Design review of the part built by this model. Coordinates are the model's own, in mm. Round coordinates to 2 decimals unless told otherwise and drop trailing zeros. One line per item, written item: value. Start each with the question number.
Item 1: We need section A-A (y = 0.9). State how many separate pieces and enclosed holes the cut face has, then the cut area to 3 significant figures.
Item 2: For line 1 along X through (y, z) = (1.3, 60); line 2 along Z through (x, y) = (-52.5, 1.05); line 3 along Z through (x, y) = (51.5, 0.1), list the stretches that pass through material, from the lowest coordinate up.
Item 3: Clearance check with a flat-ended pin moving along its axis: pin 1 (3.5 mm diameter, centred on x = 35, z = -60, fed in from -Y). State where the tip first meets the part, or that it passes through.
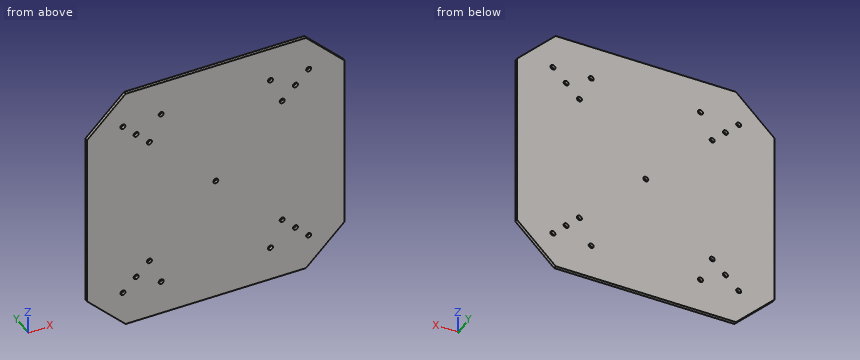
from build123d import *

# Parameters (mm, degrees)
BOSS_EXTRUDE1_DEPTH  = 2
M3_CLEARANCE_HOLE1_D = 3.2
M3_CLEARANCE_HOLE2_D = 3.2


with BuildPart() as part:
    # Sketch1 → Boss-Extrude1 (new body)
    with BuildSketch(Plane(origin=(0, 0, 0), x_dir=(1, 0, 0), z_dir=(0, 1, 0))):
        Polygon((-57.751262658, 82.5), (-82.5, 57.751262658), (-82.5, -57.751262658), (-57.751262658, -82.5), (57.751262658, -82.5), (82.5, -57.751262658), (82.5, 57.751262658), (57.751262658, 82.5), align=None)
    extrude(amount=BOSS_EXTRUDE1_DEPTH)

    # M3 Clearance Hole1 (through all)
    with Locations(Plane(origin=(0, 0, 0), x_dir=(-1, 0, 0), z_dir=(0, -1, 0))):
        with Locations((42.548466863, -42.548466863), (59.519029611, 59.519029611), (51.033748237, 51.033748237), (42.548466863, 42.548466863), (-59.519029611, -59.519029611), (-51.033748237, -51.033748237), (-42.548466863, -42.548466863), (-59.519029611, 59.519029611), (-51.033748237, 51.033748237), (-42.548466863, 42.548466863), (59.519029611, -59.519029611), (51.033748237, -51.033748237)):
            Hole(M3_CLEARANCE_HOLE1_D / 2)

    # M3 Clearance Hole2 (through all)
    with Locations(Plane(origin=(0, 2, 0), x_dir=(1, 0, 0), z_dir=(0, 1, 0))):
        with Locations((0, 0), (-35, 60), (35, -60), (35, 60), (-35, -60)):
            Hole(M3_CLEARANCE_HOLE2_D / 2)


solid = part.part
A:
1. separate pieces: 1
1. enclosed holes: 17
1. area: 25,900 mm2
2. line 1: -80.25 to -61.05, -57.99 to -36.6, -33.4 to 33.4, 36.6 to 57.99, 61.05 to 80.25
2. line 2: -82.5 to -51.67, -50.39 to 50.39, 51.67 to 82.5
2. line 3: -82.5 to -52.56, -49.5 to 49.5, 52.56 to 82.5
3. pin 1: y = 0
